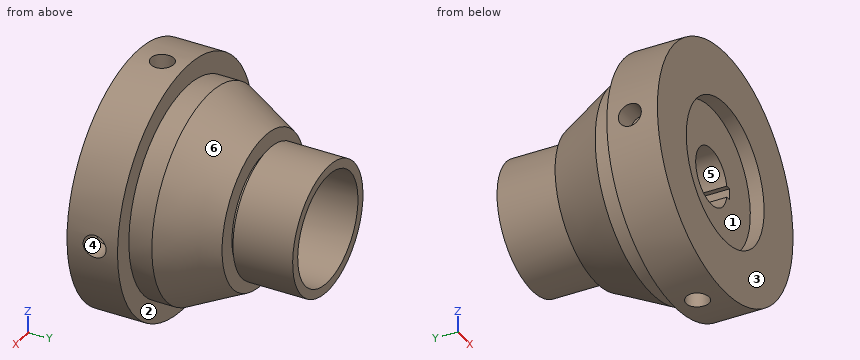
from build123d import *

# Parameters (mm, degrees)
SKETCH2_W          = 3.901140831
SKETCH2_H          = 5
CUT_EXTRUDE1_DEPTH = 99.366661019
CIRPATTERN1_COUNT  = 4


with BuildPart() as part:
    # Sketch1 → Revolve1 (revolve)
    with BuildSketch(Plane.XY, mode=Mode.PRIVATE) as revolve1_sk:
        Polygon((24, 84), (24, 62), (12.5, 62), (12.5, 6), (31, 6), (31, 0), (54, 0), (54, 22), (45, 22), (45, 32), (33, 56), (25.142857143, 56), (25.142857143, 58), (28, 58), (28, 84), align=None)
    revolve(revolve1_sk.sketch.rotate(Axis((0, 70.99827883, 0), (0, -1, 0)), 90), axis=Axis((0, 70.99827883, 0), (0, -1, 0)))

    # Sketch2 → Cut-Extrude1 (cut, through all)
    with BuildSketch(Plane(origin=(0, 62, 0), x_dir=(1, 0, 0), z_dir=(0, 1, 0))):
        with Locations((12.549429585, 0)):
            Rectangle(SKETCH2_W, SKETCH2_H)
    extrude(amount=-CUT_EXTRUDE1_DEPTH, mode=Mode.SUBTRACT)

    # Sketch10 → Ø10.0 (10) Diameter Hole1 (revolve, cut)
    with BuildSketch(Plane(origin=(-0.044253974, 12, 53.999981867), x_dir=(0.99999966419503, 0, 0.0008195180458038231), z_dir=(0, 1, 0))):
        Polygon((0, 0), (0, 13.004303095), (5, 10), (5, 0), align=None)
    f_10_0_10_diameter_hole1 = revolve(axis=Axis((-0.049457914, 12, 60.349979734), (0.000819518045803823, 0, -0.99999966419503)), mode=Mode.SUBTRACT)

    # CirPattern1: Ø10.0 (10) Diameter Hole1 ×4 about axis
    cirpattern1_axis = Axis((0, 0, 0), (0, 1, 0))
    for i in range(1, CIRPATTERN1_COUNT):
        add(f_10_0_10_diameter_hole1.rotate(cirpattern1_axis, i * 360 / CIRPATTERN1_COUNT), mode=Mode.SUBTRACT)


solid = part.part
Check sheet for the modelled part. Datum: model origin and axes. Units: mm. Face numbers are marked on the shaded views. A direction names the side the tool comes from. Coordinates: 2 decimals unless noted, no trailing zeros. Loops run counter-clockwise (first coordinate to the right, second up) from the corner with the lowest first, then second, coordinate; pieces in that order, holes last. Notation, with made-up numbers: (30, 82.5) -> (41, 82.5) arc R9 ccw to (41, 96.5) -> close; hole circle Ø10 at (89.5, 19.5). An arc over 180 degrees is marked (long way). Write item = value, one per line. Start each with the question number.
1. Section check A-A on y = 35. Record the cut outline in (x, z).
2. Material ranges on line 1 (Y direction, x = 20.5, z = 16.5); line 2 (X direction, y = 72.25, z = 0); line 3 (X direction, y = 22.5, z = 0), recorded low to high.
3. Draft check along Y on the marked faces 3, 4, 5 and 6. Enter one of: released by +Y, released by -Y, zero draft, split by the parting line, or undercut.
4. Section check C-C on y = 79. Record the cut outline in (x, z), then the cut area to 3 significant figures.
5. Depth check by flat-ended pin: P1, Ø5.5, axis at y = 21.5, z = 0.5, coming from the -X side; P2, Ø1.5, axis at x = -22, y = 16.5, coming from the -Z side; P3, Ø5, axis at x = 30, z = -37, coming from the -Y side; P4, Ø6, axis at x = -2, y = 73, coming from the +Z side. Enter the tip coordinate at first touch or a pass-through.
6. Tool access check on the marked faces 1 and 2. Record the directions out of +Z, -Z, +X, -X, +Y, -Y that give a thin tool (end or side, any length) a straight path to the whole face; none if there is none.
7. Section check B-B on y = 49. Record the cut outline in (x, z).
Responses:
q1.outline = circle Ø87 at (0, 0); hole (12.25, -2.5) -> (14.5, -2.5) -> (14.5, 2.5) -> (12.25, 2.5) arc R12.5 ccw (long way) to start
q2.line_1 = 6 to 56, 58 to 84
q2.line_2 = -28 to -24, 24 to 28
q2.line_3 = -45 to -12.5, 14.5 to 45
q3.face_3 = released by -Y
q3.face_4 = undercut
q3.face_5 = zero draft
q3.face_6 = released by +Y
q4.outline = circle Ø56 at (0, 0); hole circle Ø48 at (0, 0)
q4.area = 653 mm2
q5.P1 = -54
q5.P2 = -49.64
q5.P3 = 0
q5.P4 = 28
q6.face_1 = -Y
q6.face_2 = +Y
q7.outline = circle Ø73 at (0, 0); hole (12.25, -2.5) -> (14.5, -2.5) -> (14.5, 2.5) -> (12.25, 2.5) arc R12.5 ccw (long way) to start
